For this review, take the finished solid that the model builds, in its own axes (mm). Round coordinates to 2 decimals unless told otherwise and drop trailing zeros. Order: outer loops, then holes, each group sorted by start corner. A loop starts at its lowest first (then second) coordinate and runs counter-clockwise, first axis right, second up. Notation, with made-up numbers: M 34,26 L 46,26 A34 ccw 46,59 Z; hole C 46.25,-21.5 d5. An arc over 180 degrees is marked long. Put each result on its own line as item: value.
from build123d import *

# Parameters (mm, degrees)
CHAMFER1_SIZE = 0.275
FILLET1_R     = 0.275
FILLET2_R     = 0.1375


with BuildPart() as part:
    # Sketch3 → Revolve1 (revolve)
    with BuildSketch(Plane(origin=(0, 0, 0), x_dir=(0, 0, -1), z_dir=(1, 0, 0))):
        Polygon((4, 8), (2, 8), (2, 6.015), (-4, 6.015), (-4, 4.005), (4, 4.005), align=None)
    revolve(axis=Axis((0, 0, -4), (0, 0, 1)))

    # Chamfer1
    chamfer1_edges = [part.edges().sort_by_distance(p)[0] for p in [
        (0, -4.005, 4),
        (0, -6.015, 4),
        (0, -8, -2),
    ]]
    chamfer(chamfer1_edges, length=CHAMFER1_SIZE)

    # Fillet1
    fillet1_edges = [part.edges().sort_by_distance(p)[0] for p in [
        (0, -8, -4),
    ]]
    fillet(fillet1_edges, radius=FILLET1_R)

    # Fillet2
    fillet2_edges = [part.edges().sort_by_distance(p)[0] for p in [
        (0, -6.015, -2),
    ]]
    fillet(fillet2_edges, radius=FILLET2_R)


solid = part.part
(1) To check wall thickness, follow L1, parallel to X at y = 0, z = 1.5 (3 decimals); L2, parallel to Y at x = 0, z = -2.5 (3 decimals). State the ranges of each line that lie inside material, in increasing order.
A:
L1: x = -6.015 to -4.005, 4.005 to 6.015
L2: y = -8 to -4.005, 4.005 to 8
(2) Insertion check: pin 1 Ø4 at (y, z) = (3, -0.5) entering from +X; pin 2 Ø4 at (x, z) = (5, 0.5) entering from -Y; pin 3 Ø1 at (y, z) = (1.5, 0.5) entering from -X. Each pin has a flat end and moves straight along its axis. Give the tip position at first contact, or say it passes through.
A:
pin 1: stops at x = 7.73
pin 2: stops at y = -5.21
pin 3: stops at x = -5.93
(3) Draft analysis for pull direction Y (two halves, no side actions). For faces 1 (the face through (-1.807, 5.737, 0.97)), 2 (the face through (-1.2, 3.82, -0.19)), 3 (the face through (2, -6, -2)), state which applies: released by +Y, released by -Y, zero draft, split by the parting line, or undercut.
A:
face 1: split by the parting line
face 2: undercut
face 3: zero draft
(4) Add section C-C on z = 0.25. Give the boundary of the cut face in (x, y) (3 decimals), then the cut area to 3 significant figures.
A:
outline: C 0,0 d12.03; hole C 0,0 d8.01
area: 63.3 mm2
